```python
from build123d import *

# Parameters (mm, degrees)
BOSS_EXTRU_1_DEPTH = 6


with BuildPart() as part:
    # Esquisse1 → Boss.-Extru.1 (new body)
    with BuildSketch(Plane.XY):
        Polygon((10, 30), (17.320508076, 30), (20.980762114, 23.660254038), (26.176914536, 26.660254038), (29.176914536, 21.464101615), (23.980762114, 18.464101615), (24.980762114, 16.732050808), (22.382685902, 15.232050808), (21.607685902, 16.574390183), (18.92300715, 15.024390183), (19.69800715, 13.682050808), (16.320508076, 11.732050808), (18.320508076, 8.267949192), (21.69800715, 10.217949192), (22.47300715, 8.875609817), (25.157685902, 10.425609817), (24.382685902, 11.767949192), (26.980762114, 13.267949192), (27.980762114, 11.535898385), (33.176914536, 14.535898385), (36.176914536, 9.339745962), (30.980762114, 6.339745962), (34.641016151, 0), (30.980762114, -6.339745962), (36.176914536, -9.339745962), (33.176914536, -14.535898385), (27.980762114, -11.535898385), (26.980762114, -13.267949192), (24.382685902, -11.767949192), (25.182685902, -10.382308546), (22.41140461, -8.782308546), (21.61140461, -10.167949192), (18.320508076, -8.267949192), (16.320508076, -11.732050808), (19.61140461, -13.632050808), (18.81140461, -15.017691454), (21.582685902, -16.617691454), (22.382685902, -15.232050808), (24.980762114, -16.732050808), (23.980762114, -18.464101615), (29.176914536, -21.464101615), (26.176914536, -26.660254038), (20.980762114, -23.660254038), (17.320508076, -30), (10, -30), (10, -36), (4, -36), (4, -30), (2, -30), (2, -27), (3.65, -27), (3.65, -23.7), (2, -23.7), (2, -20), (-2, -20), (-2, -23.7), (-3.65, -23.7), (-3.65, -27), (-2, -27), (-2, -30), (-4, -30), (-4, -36), (-10, -36), (-10, -30), (-14, -30), (-14, 30), (-10, 30), (-10, 36), (-4, 36), (-4, 30), (-2, 30), (-2, 27), (-3.5, 27), (-3.5, 24), (-2, 24), (-2, 20), (2, 20), (2, 24), (3.5, 24), (3.5, 27), (2, 27), (2, 30), (4, 30), (4, 36), (10, 36), align=None)
    extrude(amount=BOSS_EXTRU_1_DEPTH)


solid = part.part
```
The model under review builds one solid part; all positions refer to its coordinate system, in mm. A direction names the side the tool comes from. Round coordinates to 2 decimals unless told otherwise and drop trailing zeros. Loops run counter-clockwise (first coordinate to the right, second up) from the corner with the lowest first, then second, coordinate; pieces in that order, holes last.
1) The part is to be moulded in two halves that separate along X. For faces 1 (the face through (-3, -30, 3)), 2 (the face through (-14, 0, 3)), 3 (the face through (7, 36, 3)), say which applies: pulls with the +X half, pulls with the -X half, needs draft (parallel to the pull), parting line crosses it, or undercut.
Values follow:
face 1: undercut
face 2: pulls with the -X half
face 3: needs draft
2) Wall thickness on line 1 along Y through (x, z) = (33, 3.2); line 2 along Y through (x, z) = (21, 1.6); line 3 along X through (y, z) = (10, 1.7): over which ranges is each line inside the solid? List them lowest first.
Values follow:
line 1: y = -14.43 to -7.51, -2.84 to 2.84, 7.51 to 14.43
line 2: y = -23.67 to -16.28, -9.81 to 9.81, 16.22 to 23.67
line 3: x = -14 to 17.32, 21.32 to 21.82, 24.42 to 35.8
3) Consider section A-A on y = 28.5. State the section outline as (x, z) points, then the cut area to 3 significant figures.
Values follow:
outline: (-14, 0) - (-2, 0) - (-2, 6) - (-14, 6) - close; (2, 0) - (18.19, 0) - (18.19, 6) - (2, 6) - close
area: 169 mm2
4) Consider section C-C on x = 14. State the section outline as (y, z) points, then the cut area to 3 significant figures.
Values follow:
outline: (-30, 0) - (30, 0) - (30, 6) - (-30, 6) - close
area: 360 mm2
5) Clearance check with flat-ended pins moving along their axes: P1, Ø1.6, axis at x = -2.5, z = 3.5, coming from the +Y side; P2, Ø1, axis at x = 2.5, z = 2, coming from the -Y side; P3, Ø3.5, axis at y = 26, z = 4.5, coming from the +X side. State where each tip first meets the part, or that it passes through.
Values follow:
P1: stops at y = 30
P2: stops at y = -30
P3: stops at x = 27.57
6) Tool access review of faces 4 (the face through (-3, 30, 3)), 5 (the face through (26.62, 19.99, 2.96)), 6 (the face through (-12, -30, 3)), 7 (the face through (17.943, -12.669, 2.958)), 8 (the face through (0, -20, 3)): name each direction out of +Z, -Z, +X, -X, +Y, -Y from which nothing blocks a thin tool from reaching the whole face with its end or side.
Values follow:
face 4: +Z, -Z, +Y
face 5: +Z, -Z, +X
face 6: +Z, -Z, -X, -Y
face 7: +Z, -Z
face 8: +Z, -Z, -Y
7) Consider section B-B on y = -24.5. State the section outline as (x, z) points, then the cut area to 3 significant figures.
Values follow:
outline: (-14, 0) - (-3.65, 0) - (-3.65, 6) - (-14, 6) - close; (3.65, 0) - (20.5, 0) - (20.5, 6) - (3.65, 6) - close; (22.44, 0) - (27.42, 0) - (27.42, 6) - (22.44, 6) - close
area: 193 mm2
